CAD build for the part. Positions are in the model's coordinates, mm. Give positions to 0.01 mm unless a question says otherwise; leave off trailing zeros. Write each loop counter-clockwise with the first axis right and the second up, starting at its lowest first coordinate (ties: lowest second). Pieces come first, ordered by that corner, then holes. Notation, with made-up numbers: (14.25, -38.75) - (57.25, -38.75) arc R21 cw to (57.25, -3.75) - close; hole circle Ø6 at (11.25, 83.25). An arc over 180 degrees is marked (long way). Answer as a JSON object with one key per item and string values.
from build123d import *

# Parameters (mm, degrees)
BOSS_EXTRUDE1_DEPTH  = 147
FILLET1_R            = 18.5
CUT_EXTRUDE1_DEPTH   = 50
FILLET2_R            = 20
FILLET1_OF_MIRROR1_R = 18.5
FILLET2_OF_MIRROR1_R = 20


with BuildPart() as part:
    # Sketch1 → Boss-Extrude1 (new body)
    with BuildSketch(Plane(origin=(0, 0, 0), x_dir=(1, 0, 0), z_dir=(0, 1, 0))):
        Polygon((-73.50000000000001, 73.5), (73.5, 73.49999999999999), (73.50000000000001, 0), (-73.50000000000001, 0), align=None)
    boss_extrude1 = extrude(amount=BOSS_EXTRUDE1_DEPTH)

    # Fillet1
    fillet1_edges = [part.edges().sort_by_distance(p)[0] for p in [
        (73.5, 147, -36.74999999999999),
        (-1.421e-14, 147, -73.5),
        (-73.50000000000001, 147, -36.75),
        (-1.421e-14, 0, -73.5),
        (73.5, 0, -36.74999999999999),
        (-73.50000000000001, 0, -36.75),
        (-73.50000000000001, 73.5, -73.5),
        (73.5, 73.5, -73.49999999999999),
    ]]
    fillet(fillet1_edges, radius=FILLET1_R)

    # Sketch2 → Cut-Extrude1 (cut)
    with BuildSketch(Plane.XY):
        Polygon((-50.00000000000003, 137), (49.99999999999997, 137.00000000000006), (50.00000000000007, 2.000000000000012), (-50.00000000000004, 2), align=None)
    cut_extrude1 = extrude(amount=-CUT_EXTRUDE1_DEPTH, mode=Mode.SUBTRACT)

    # Fillet2
    fillet2_edges = [part.edges().sort_by_distance(p)[0] for p in [
        (-50.000000000000036, 69.5, -50),
        (-50.00000000000004, 2, -25),
        (-2.842e-14, 137.00000000000003, -50),
        (-50.00000000000003, 137, -25),
        (50.00000000000002, 69.50000000000003, -50),
        (49.99999999999997, 137.00000000000006, -25),
        (1.421e-14, 2.000000000000006, -50),
        (50.00000000000007, 2.000000000000012, -25),
    ]]
    fillet(fillet2_edges, radius=FILLET2_R)

    # Mirror1: Boss-Extrude1, Cut-Extrude1 across plane
    add(boss_extrude1.mirror(Plane(origin=(-73.50000000000001, 147, 0), x_dir=(1, 0, 0), z_dir=(0, 0, -1))))
    add(cut_extrude1.mirror(Plane(origin=(-73.50000000000001, 147, 0), x_dir=(1, 0, 0), z_dir=(0, 0, -1))), mode=Mode.SUBTRACT)

    # Fillet1 of Mirror1
    fillet1_of_mirror1_edges = [part.edges().sort_by_distance(p)[0] for p in [
        (73.5, 147, 36.74999999999999),
        (-1.421e-14, 147, 73.5),
        (-73.50000000000001, 147, 36.75),
        (-1.421e-14, 0, 73.5),
        (73.5, 0, 36.74999999999999),
        (-73.50000000000001, 0, 36.75),
        (-73.50000000000001, 73.5, 73.5),
        (73.5, 73.5, 73.49999999999999),
    ]]
    fillet(fillet1_of_mirror1_edges, radius=FILLET1_OF_MIRROR1_R)

    # Fillet2 of Mirror1
    fillet2_of_mirror1_edges = [part.edges().sort_by_distance(p)[0] for p in [
        (-50.000000000000036, 69.5, 50),
        (-50.00000000000004, 2, 25),
        (-2.842e-14, 137.00000000000003, 50),
        (-50.00000000000003, 137, 25),
        (50.00000000000002, 69.50000000000003, 50),
        (49.99999999999997, 137.00000000000006, 25),
        (1.421e-14, 2.000000000000006, 50),
        (50.00000000000007, 2.000000000000012, 25),
    ]]
    fillet(fillet2_of_mirror1_edges, radius=FILLET2_OF_MIRROR1_R)


solid = part.part
Item 1: Mould opens along Z. For faces 1 (the cylindrical face through (0.77, 141.44, -68.22)), 2 (the cylindrical face through (68.22, 5.56, -27.11)), 3 (the flat face through (0, 137, 0)), 4 (the cylindrical face through (0.77, 141.44, 68.22)) say: +Z half, -Z half, draft (parallel to the pull), parting line (faces both ways), or undercut.
Entries:
{"face 1": "-Z half", "face 2": "draft", "face 3": "undercut", "face 4": "+Z half"}
Item 2: Probe line 1 (X direction, y = 44, z = 28.5); line 2 (Y direction, x = -31, z = -1.5). List the from-to ranges inside material, lowest first. Write a range as from..to.
Entries:
{"line 1": "-73.5..-50, 50..73.5", "line 2": "0..2.03, 136.97..147"}
Item 3: Flat gauge pins, fed straight in: P1, Ø6, axis at y = 93, z = -57, coming from the +X side; P2, Ø6, axis at x = -41, y = 14, coming from the +Z side; P3, Ø15, axis at x = 64.5, y = 12.5, coming from the -Z side. Where does each tip first touch, or does it go through?
Entries:
{"P1": "x = 73.5", "P2": "z = 73.44", "P3": "z = -73.12"}
Item 4: Cut at A-A (x = 22.5). Give the cut face in (y, z), and give its area (3 significant figures).
Entries:
{"outline": "(0, -55) arc R18.5 ccw to (18.5, -73.5) - (128.5, -73.5) arc R18.5 ccw to (147, -55) - (147, 55) arc R18.5 ccw to (128.5, 73.5) - (18.5, 73.5) arc R18.5 ccw to (0, 55) - close; hole (2, -30) arc R20 ccw to (22, -50) - (117, -50) arc R20 ccw to (137, -30) - (137, 30) arc R20 ccw to (117, 50) - (22, 50) arc R20 ccw to (2, 30) - close", "area": "8,160 mm2"}
Item 5: Cut at D-D (z = 59). Give the cut face in (x, y).
Entries:
{"outline": "(-73.06, 18.5) arc R18.06 ccw to (-55, 0.44) - (55, 0.44) arc R18.06 ccw to (73.06, 18.5) - (73.06, 128.5) arc R18.06 ccw to (55, 146.56) - (-55, 146.56) arc R18.06 ccw to (-73.06, 128.5) - close"}
Item 6: Cut at B-B (z = 11). Give the cut face in (x, y), and give its area (3 significant figures).
Entries:
{"outline": "(-73.5, 18.5) arc R18.5 ccw to (-55, 0) - (55, 0) arc R18.5 ccw to (73.5, 18.5) - (73.5, 128.5) arc R18.5 ccw to (55, 147) - (-55, 147) arc R18.5 ccw to (-73.5, 128.5) - close; hole (-50, 22) arc R20 ccw to (-30, 2) - (30, 2) arc R20 ccw to (50, 22) - (50, 117) arc R20 ccw to (30, 137) - (-30, 137) arc R20 ccw to (-50, 117) - close", "area": "8,160 mm2"}
Item 7: Cut at C-C (x = 60). Give the cut face in (y, z).
Entries:
{"outline": "(0.69, -55) arc R17.81 ccw to (18.5, -72.81) - (128.5, -72.81) arc R17.81 ccw to (146.31, -55) - (146.31, 55) arc R17.81 ccw to (128.5, 72.81) - (18.5, 72.81) arc R17.81 ccw to (0.69, 55) - close"}
